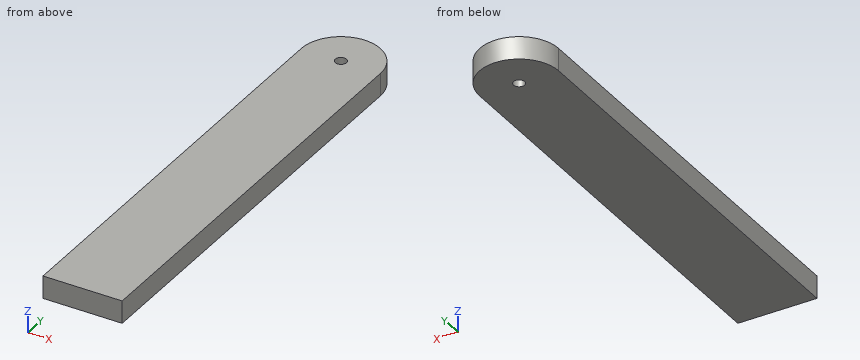
from build123d import *

# Parameters (mm, degrees)
SKETCH1_R           = 4.7625
BOSS_EXTRUDE1_DEPTH = 9.525


with BuildPart() as part:
    # Sketch1 → Boss-Extrude1 (new body, symmetric)
    with BuildSketch(Plane.XY):
        with BuildLine():
            Line((33.3375, -198.4375), (-33.3375, -198.4375))
            Line((-33.3375, -198.4375), (-33.3375, 165.1))
            ThreePointArc((-33.3375, 165.1), (0, 198.4375), (33.3375, 165.1))
            Line((33.3375, 165.1), (33.3375, -198.4375))
        make_face()
        with Locations((0, 165.1)):
            Circle(SKETCH1_R, mode=Mode.SUBTRACT)
    extrude(amount=BOSS_EXTRUDE1_DEPTH, both=True)


solid = part.part
Here's how the part is built. I have some questions about the finished solid (model axes, mm). Coordinates: 2 decimals unless noted, no trailing zeros. Order: outer loops, then holes, each group sorted by start corner. A loop starts at its lowest first (then second) coordinate and runs counter-clockwise, first axis right, second up.
Item 1: If we section it at C-C on x = -26.5: List the corners of the cut face in (y, z) for me (1 decimal).
Result sheet:
outline: (-198.4, -9.5) - (185.3, -9.5) - (185.3, 9.5) - (-198.4, 9.5) - close
Item 2: If we section it at A-A on x = 0: List the corners of the cut face in (y, z) for me (1 decimal).
Result sheet:
outline: (-198.4, -9.5) - (160.3, -9.5) - (160.3, 9.5) - (-198.4, 9.5) - close; (169.9, -9.5) - (198.4, -9.5) - (198.4, 9.5) - (169.9, 9.5) - close
Item 3: For P1, Ø8, axis at x = -10.5, z = 5, coming from the +Y side; P2, Ø8.5, axis at x = 0, y = 165.1, coming from the -Z side (1 decimal); P3, Ø5, axis at x = -21.5, z = 3.5, coming from the +Y side, each with a flat end and sliding along its axis, tell me the tip position at first contact or that it passes through.
Result sheet:
P1: stops at y = 197.8
P2: passes through
P3: stops at y = 192.49
Item 4: If we section it at B-B on z = 4.75: List the corners of the cut face in (x, y) for me (1 decimal).
Result sheet:
outline: (-33.3, -198.4) - (33.3, -198.4) - (33.3, 165.1) arc R33.3 ccw to (-33.3, 165.1) - close; hole circle Ø9.5 at (0, 165.1)
Item 5: I need wall thicknesses on line 1 (Y direction, x = 0, z = -4.75); line 2 (Y direction, x = 3, z = -5); line 3 (Y direction, x = 28, z = 4.75). Which ranges of each line are inside material? Lowest first, please.
Result sheet:
line 1: y = -198.44 to 160.34, 169.86 to 198.44
line 2: y = -198.44 to 161.4, 168.8 to 198.3
line 3: y = -198.44 to 183.19
